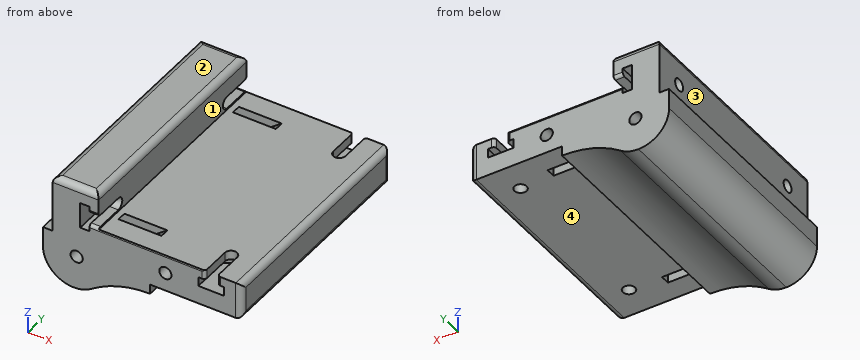
from build123d import *

# Parameters (mm, degrees)
BOSS_EXTRUDE1_DEPTH = 75
SKETCH2_R           = 2
CUT_EXTRUDE1_DEPTH  = 15
SKETCH4_R           = 2
CUT_EXTRUDE2_DEPTH  = 12
SKETCH3_R           = 2
CUT_EXTRUDE3_DEPTH  = 75
CUT_EXTRUDE4_START  = -3
CUT_EXTRUDE4_DEPTH  = 3
CUT_EXTRUDE5_START  = -3
CUT_EXTRUDE5_DEPTH  = 3
CUT_EXTRUDE6_START  = -3
CUT_EXTRUDE6_DEPTH  = 3
CUT_EXTRUDE7_START  = -3
CUT_EXTRUDE7_DEPTH  = 3
CUT_EXTRUDE8_START  = -7
CUT_EXTRUDE8_DEPTH  = 3
FILLET2_START       = 5.175
FILLET2_DEPTH       = 42.1845
FILLET2_START_2     = 10.175
FILLET2_2_DEPTH     = 3.491666667
FILLET2_3_DEPTH     = 37.825
FILLET3_R           = 2


with BuildPart() as part:
    # Sketch1 → Boss-Extrude1 (new body)
    with BuildSketch(Plane(origin=(0, 0, 0), x_dir=(1, 0, 0), z_dir=(0, 1, 0))):
        with BuildLine():
            Line((-6.825, -6.666666667), (-6.825, -25.333333333))
            Line((-6.825, -25.333333333), (8.175, -25.333333333))
            Line((8.175, -25.333333333), (8.175, -13.175))
            Line((8.175, -13.175), (55, -13.175))
            Line((55, -13.175), (55, -1.175))
            Line((55, -1.175), (25, -1.175))
            Line((25, -1.175), (25, 2))
            ThreePointArc((25, 2), (14.923352523, 3.572976633), (5.805515239, 8.142235123))
            ThreePointArc((5.805515239, 8.142235123), (3.047757271, 9.524241472), (0, 10))
            ThreePointArc((0, 10), (-7.071067812, 7.071067812), (-10, 0))
            Line((-10, 0), (-10, -6.666666667))
            Line((-10, -6.666666667), (-6.825, -6.666666667))
        make_face()
    extrude(amount=BOSS_EXTRUDE1_DEPTH)

    # Sketch2 → Cut-Extrude1 (cut)
    with BuildSketch(Plane.ZY.offset(6.825)):
        with Locations((15.666666667, 65)):
            Circle(SKETCH2_R)
    cut_extrude1 = extrude(amount=-CUT_EXTRUDE1_DEPTH, mode=Mode.SUBTRACT)

    # Sketch4 → Cut-Extrude2 (cut)
    with BuildSketch(Plane(origin=(0, 0, 1.175), x_dir=(-1, 0, 0), z_dir=(0, 0, -1))):
        with Locations((-45, 65)):
            Circle(SKETCH4_R)
    cut_extrude2 = extrude(amount=-CUT_EXTRUDE2_DEPTH, mode=Mode.SUBTRACT)

    # Sketch3 → Cut-Extrude3 (cut)
    with BuildSketch(Plane(origin=(0, 75, 0), x_dir=(1, 0, 0), z_dir=(0, 1, 0))):
        with Locations(Location((1, -1, 0), (0, 0, 270))):
            Circle(SKETCH3_R)
        with Locations(Location((30, -7.175, 0), (0, 0, 270))):
            Circle(SKETCH3_R)
    extrude(amount=-CUT_EXTRUDE3_DEPTH, mode=Mode.SUBTRACT)

    # Sketch5 → Cut-Extrude4 (cut)
    with BuildSketch(Plane(origin=(8.175, 0, 0), x_dir=(0, 0, -1), z_dir=(1, 0, 0)).offset(CUT_EXTRUDE4_START)):
        Polygon((-19.885416667, 62.564303552), (-15.666666667, 60.128607104), (-11.447916667, 62.564303552), (-11.447916667, 75), (-19.885416667, 75), align=None)
    cut_extrude4 = extrude(amount=-CUT_EXTRUDE4_DEPTH, mode=Mode.SUBTRACT)

    # Sketch6 → Cut-Extrude5 (cut)
    with BuildSketch(Plane(origin=(8.175, 0, 0), x_dir=(0, 0, -1), z_dir=(1, 0, 0)).offset(CUT_EXTRUDE5_START)):
        with BuildLine():
            Line((-13.666666667, 65), (-13.666666667, 75))
            Line((-13.666666667, 75), (-17.666666667, 75))
            Line((-17.666666667, 75), (-17.666666667, 65))
            ThreePointArc((-17.666666667, 65), (-15.666666667, 67), (-13.666666667, 65))
        make_face()
    cut_extrude5 = extrude(amount=CUT_EXTRUDE5_DEPTH, mode=Mode.SUBTRACT)

    # Sketch7 → Cut-Extrude6 (cut)
    with BuildSketch(Plane.XY.offset(13.175).offset(CUT_EXTRUDE6_START)):
        Polygon((40.78125, 62.564303552), (45, 60.128607104), (49.21875, 62.564303552), (49.21875, 75), (40.78125, 75), align=None)
    cut_extrude6 = extrude(amount=-CUT_EXTRUDE6_DEPTH, mode=Mode.SUBTRACT)

    # Sketch8 → Cut-Extrude7 (cut)
    with BuildSketch(Plane.XY.offset(13.175).offset(CUT_EXTRUDE7_START)):
        with BuildLine():
            Line((47, 65), (47, 75))
            Line((47, 75), (43, 75))
            Line((43, 75), (43, 65))
            ThreePointArc((43, 65), (45, 67), (47, 65))
        make_face()
    cut_extrude7 = extrude(amount=CUT_EXTRUDE7_DEPTH, mode=Mode.SUBTRACT)

    # Sketch10 → Cut-Extrude8 (cut)
    with BuildSketch(Plane(origin=(0, 75, 0), x_dir=(1, 0, 0), z_dir=(0, 1, 0)).offset(CUT_EXTRUDE8_START)):
        Polygon((0.411941919, -5.835768444), (10.175, -13.175), (24.216737808, -13.175), (5.48192736, 0.908610985), (1.588058081, 3.835768444), (-2.893869279, 1.927157459), (-3.48192736, -2.908610985), align=None)
        Polygon((25.78125, -4.739303552), (25.78125, -1.175), (34.21875, -1.175), (34.21875, -4.739303552), (34.21875, -9.610696448), (30, -12.046392896), (25.78125, -9.610696448), align=None)
    cut_extrude8 = extrude(amount=-CUT_EXTRUDE8_DEPTH, mode=Mode.SUBTRACT)

    # Mirror2: Cut-Extrude1, Cut-Extrude2, Cut-Extrude4, Cut-Extrude5, Cut-Extrude6, Cut-Extrude7, Cut-Extrude8 across plane
    add(cut_extrude1.mirror(Plane.ZX.offset(37.5)), mode=Mode.SUBTRACT)
    add(cut_extrude2.mirror(Plane.ZX.offset(37.5)), mode=Mode.SUBTRACT)
    add(cut_extrude4.mirror(Plane.ZX.offset(37.5)), mode=Mode.SUBTRACT)
    add(cut_extrude5.mirror(Plane.ZX.offset(37.5)), mode=Mode.SUBTRACT)
    add(cut_extrude6.mirror(Plane.ZX.offset(37.5)), mode=Mode.SUBTRACT)
    add(cut_extrude7.mirror(Plane.ZX.offset(37.5)), mode=Mode.SUBTRACT)
    add(cut_extrude8.mirror(Plane.ZX.offset(37.5)), mode=Mode.SUBTRACT)

    # Fillet2: read off the stored shape, not the designer's step
    # Fillet2 outline → Fillet2 (cut)
    with BuildSketch(Plane.YZ.offset(FILLET2_START)):
        with BuildLine():
            Line((1, 13.666666667), (0, 13.666666667))
            Line((0, 13.666666667), (0, 12.666666667))
            ThreePointArc((0, 12.666666667), (0.292893219, 13.373773448), (1, 13.666666667))
        make_face()
        with BuildLine():
            ThreePointArc((1, 17.666666667), (0.292893218, 17.959559886), (0, 18.666666667))
            Line((0, 18.666666667), (0, 17.666666667))
            Line((0, 17.666666667), (1, 17.666666667))
        make_face()
    extrude(amount=FILLET2_DEPTH, mode=Mode.SUBTRACT)

    # Fillet2 2 outline → Fillet2 2 (cut)
    with BuildSketch(Plane.XY.offset(FILLET2_START_2)):
        with BuildLine():
            Line((47, 1), (47, 0))
            Line((47, 0), (47.3595, 0))
            Line((47.3595, 0), (48, 0))
            ThreePointArc((48, 0), (47.292893219, 0.292893219), (47, 1))
        make_face()
        with BuildLine():
            Line((48, 75), (47, 75))
            Line((47, 75), (47, 74))
            ThreePointArc((47, 74), (47.292893219, 74.707106781), (48, 75))
        make_face()
        with BuildLine():
            Line((43, 75), (42, 75))
            ThreePointArc((42, 75), (42.707106781, 74.707106781), (43, 74))
            Line((43, 74), (43, 75))
        make_face()
        with BuildLine():
            ThreePointArc((43, 1), (42.707106781, 0.292893219), (42, 0))
            Line((42, 0), (43, 0))
            Line((43, 0), (43, 1))
        make_face()
    extrude(amount=FILLET2_2_DEPTH, mode=Mode.SUBTRACT)

    # Fillet2 3 outline → Fillet2 3 (cut)
    with BuildSketch(Plane.YZ.offset(FILLET2_START)):
        with BuildLine():
            Line((74, 17.666666667), (75, 17.666666667))
            Line((75, 17.666666667), (75, 18.666666667))
            ThreePointArc((75, 18.666666667), (74.707106782, 17.959559886), (74, 17.666666667))
        make_face()
        with BuildLine():
            Line((75, 12.666666667), (75, 13.666666667))
            Line((75, 13.666666667), (74, 13.666666667))
            ThreePointArc((74, 13.666666667), (74.707106781, 13.373773448), (75, 12.666666667))
        make_face()
    extrude(amount=FILLET2_3_DEPTH, mode=Mode.SUBTRACT)

    # Fillet3
    fillet3_edges = [part.edges().sort_by_distance(p)[0] for p in [
        (55, 0, 7.175),
        (0.675, 0, 25.333333333),
        (55, 37.5, 1.175),
        (55, 37.5, 13.175),
        (8.175, 37.5, 25.333333333),
        (-6.825, 37.5, 25.333333333),
        (0.675, 75, 25.333333333),
        (55, 75, 7.175),
    ]]
    fillet(fillet3_edges, radius=FILLET3_R)


solid = part.part
Could you check a few things on this model? Use its own coordinates, in mm. Face numbers are marked on the shaded views. A direction names the side the tool comes from. Coordinates: 2 decimals unless noted, no trailing zeros. Order: outer loops, then holes, each group sorted by start corner. A loop starts at its lowest first (then second) coordinate and runs counter-clockwise, first axis right, second up. Notation, with made-up numbers: (34.5, -27.5) -> (91.5, -27.5) arc R26 ccw to (91.5, -0.5) -> close; hole circle Ø8 at (22.25, -4.5). An arc over 180 degrees is marked (long way). One line per item, written item: value. Start each with the question number.
1) If I drill on L1, parallel to Y at x = 4, z = 1.5; L2, parallel to X at y = 30, z = 1; L3, parallel to Z at x = 51.5, y = 22 (3 decimals), over which ranges is the centre line in solid material (lowest first)? Write a range as [from, to].
2) Imagine slicing it at A-A on y = 42. List the corners of the cut face in (x, z) for me (1 decimal), plus the area to 3 significant figures.
3) Imagine slicing it at C-C on z = 21.5. List the corners of the cut face in (x, y) for me (3 decimals), plus the area to 4 significant figures.
4) Imagine slicing it at D-D on y = 70. Count the separate pieces of the cut face and the enclosed holes in it, plus the area to 3 significant figures.
5) Imagine slicing it at B-B on x = 16. List the corners of the cut face in (y, z) for me (3 decimals).
6) I'm going to push flat-ended pins straight in: pin 1 (6 mm diameter, centred on y = 40, z = 18.5, fed in from -X) (3 decimals); pin 2 (1.5 mm diameter, centred on x = 16, y = 59.5, fed in from -Z); pin 3 (4.5 mm diameter, centred on y = 10, z = 15.67, fed in from +X) (3 decimals). Where does each tip first touch, or does it pass through?
7) Which directions (+Z, -Z, +X, -X, +Y, -Y) give clear straight access to the entire face, cutting with the end or side of a thin tool? Please do the marked faces 1, 2, 3 and 4.
Answer list:
1. L1: y = [0, 7], [10, 65], [68, 75]
1. L2: x = [-10, -1], [3, 25]
1. L3: z = [1.175, 13.175]
2. outline: (-10, 0) arc R10 ccw to (5.8, -8.1) arc R33.1 cw to (25, -2) -> (25, 1.2) -> (53, 1.2) arc R2 ccw to (55, 3.2) -> (55, 11.2) arc R2 ccw to (53, 13.2) -> (8.2, 13.2) -> (8.2, 23.3) arc R2 ccw to (6.2, 25.3) -> (-4.8, 25.3) arc R2 ccw to (-6.8, 23.3) -> (-6.8, 6.7) -> (-10, 6.7) -> close; hole circle Ø4 at (1, 1); hole circle Ø4 at (30, 7.2)
2. area: 1,160 mm2
3. outline: (-6.825, 0) -> (8.175, 0) -> (8.175, 75) -> (-6.825, 75) -> close
3. area: 1,125 mm2
4. separate pieces: 1
4. enclosed holes: 2
4. area: 1,090 mm2
5. outline: (0, -3.249) -> (75, -3.249) -> (75, 12.667) arc R1 ccw to (74.861, 13.175) -> (68, 13.175) -> (68, 6.998) -> (65, 6.998) -> (65, 13.175) -> (10, 13.175) -> (10, 6.998) -> (7, 6.998) -> (7, 13.175) -> (0.139, 13.175) arc R1 ccw to (0, 12.667) -> close
6. pin 1: stops at x = -6.825
6. pin 2: stops at z = -3.47
6. pin 3: stops at x = 8.175
7. face 1: +Z, +X, +Y, -Y
7. face 2: +Z, +X, -X, +Y, -Y
7. face 3: +Z, -X, +Y, -Y
7. face 4: -Z, +X, +Y, -Y
